```python
from build123d import *

# Parameters (mm, degrees)
PAD_DEPTH           = 110
PAD001_DEPTH        = 96
SKETCH003_W         = 118.6
SKETCH003_H         = 10
PAD002_DEPTH        = 3
PAD003_DEPTH        = 123
POCKET001_DEPTH     = 124.601
LINEARPATTERN_COUNT = 5
LINEARPATTERN_PITCH = 22.5
SKETCH012_W         = 6
SKETCH012_H         = 12
POCKET_DEPTH        = 5
SKETCH013_R         = 1.7
POCKET004_DEPTH     = 126.001
SKETCH014_R         = 7
SKETCH014_R_2       = 2
POCKET005_DEPTH     = 5


with BuildPart() as part:
    # Sketch → Pad (new body)
    with BuildSketch(Plane.XY):
        Polygon((62.3, 64.5), (-62.3, 64.5), (-62.3, -61.5), (-59.3, -61.5), (-59.3, 61.5), (59.3, 61.5), (59.3, -61.5), (62.3, -61.5), align=None)
    extrude(amount=PAD_DEPTH)

    # Sketch001 → Pad001 (join)
    with BuildSketch(Plane.XY):
        Polygon((-59.3, 59.5), (-57.3, 61.5), (-59.3, 61.5), align=None)
    pad001 = extrude(amount=PAD001_DEPTH)

    # Mirrored: Pad001 across YZ
    add(pad001.mirror(Plane.YZ))

    # Sketch003 (on DatumPlane) → Pad002 (join)
    with BuildSketch(Plane.XZ.offset(61.5)):
        with Locations((0, 5)):
            Rectangle(SKETCH003_W, SKETCH003_H)
    extrude(amount=-PAD002_DEPTH)

    # Sketch004 (on DatumPlane) → Pad003 (join)
    with BuildSketch(Plane.XZ.offset(61.5)):
        Polygon((-57.3, 117), (-59.3, 117), (-59.3, 100), (-57.3, 103), align=None)
        Polygon((57.3, 103), (57.3, 117), (59.3, 117), (59.3, 100), align=None)
    extrude(amount=-PAD003_DEPTH)

    # Sketch009 (on DatumPlane) → Pocket001 (cut, through all)
    with BuildSketch(Plane.YZ.offset(62.3)):
        with BuildLine():
            Line((-46, 20), (-46, 243))
            ThreePointArc((-42, 243), (-44, 245), (-46, 243))
            Line((-42, 243), (-42, 20))
            ThreePointArc((-46, 20), (-44, 18), (-42, 20))
        make_face()
    pocket001 = extrude(amount=-POCKET001_DEPTH, mode=Mode.SUBTRACT)

    # LinearPattern: Pocket001 ×5
    with Locations(*[(0, i * LINEARPATTERN_PITCH, 0) for i in range(1, LINEARPATTERN_COUNT)]):
        add(pocket001, mode=Mode.SUBTRACT)

    # Sketch012 (on DatumPlane) → Pocket (cut)
    with BuildSketch(Plane.YZ.offset(62.3)):
        with Locations((41.830656, 89.723986)):
            Rectangle(SKETCH012_W, SKETCH012_H)
        with Locations((41.830656, 62.651357)):
            Rectangle(SKETCH012_W, SKETCH012_H)
    extrude(amount=-POCKET_DEPTH, mode=Mode.SUBTRACT)

    # Sketch013 (on DatumPlane) → Pocket004 (cut, through all)
    with BuildSketch(Plane.XZ.offset(-64.5)):
        with Locations((20, 5)):
            Circle(SKETCH013_R)
        with Locations((-20, 5)):
            Circle(SKETCH013_R)
    extrude(amount=POCKET004_DEPTH, mode=Mode.SUBTRACT)

    # Sketch014 (on DatumPlane) → Pocket005 (cut)
    with BuildSketch(Plane.XZ.offset(-64.5)):
        with Locations((-16.307726, 38.976202)):
            Circle(SKETCH014_R)
        with Locations((-41.75, 38.976202)):
            Circle(SKETCH014_R)
        with Locations((-44.911871, 102.251883)):
            Circle(SKETCH014_R_2)
        Polygon((32, 0), (52, 0), (52, 18), (42, 28), (32, 18), align=None)
        Polygon((-52, 0), (-32, 0), (-32, 18), (-42, 28), (-52, 18), align=None)
    extrude(amount=POCKET005_DEPTH, mode=Mode.SUBTRACT)


with BuildPart() as part_1:
    # Body placement: moved
    add(part.part.moved(Location((1.4, 0, 0))))


solid = part_1.part
```
CAD build for the part. Positions are in the model's coordinates, mm. A direction names the side the tool comes from. Give positions to 0.01 mm unless a question says otherwise; leave off trailing zeros. Loops run counter-clockwise (first coordinate to the right, second up) from the corner with the lowest first, then second, coordinate; pieces in that order, holes last. Notation, with made-up numbers: (-2, -36.75) -> (25, -36.75) arc R26 ccw to (25, -15.75) -> close; hole circle Ø5 at (-35.75, 3). An arc over 180 degrees is marked (long way). Use a Markdown table: item, result.
1. Flat gauge pins, fed straight in: pin 1 (0.9 mm diameter, centred on x = -60, y = -13.5, fed in from +Z); pin 2 (1.5 mm diameter, centred on x = -7, y = -59.5, fed in from +Z); pin 3 (3 mm diameter, centred on x = -43.51, z = 102.25, fed in from +Y). Where does each tip first touch, or does it go through?
Check result:
| item | result |
|---|---|
| pin 1 | stops at z = 110 |
| pin 2 | stops at z = 10 |
| pin 3 | passes through |
2. Slice it at C-C (z = 5). Give the number of separate pieces and of enclosed holes in the cut face, plus the area to 3 significant figures.
Check result:
| item | result |
|---|---|
| separate pieces | 6 |
| enclosed holes | 0 |
| area | 1,310 mm^2 |
3. Slice it at D-D (x = -14). List the corners of the cut face in (y, z).
Check result:
| item | result |
|---|---|
| outline | (-61.5, 0) -> (-58.5, 0) -> (-58.5, 10) -> (-61.5, 10) -> close; (61.5, 0) -> (64.5, 0) -> (64.5, 32.04) -> (61.5, 32.04) -> close; (61.5, 45.92) -> (64.5, 45.92) -> (64.5, 110) -> (61.5, 110) -> close |
4. Slice it at A-A (y = 41). List the corners of the cut face in (x, z), plus the area to 3 significant figures.
Check result:
| item | result |
|---|---|
| outline | (-60.9, 0) -> (-57.9, 0) -> (-57.9, 100) -> (-55.9, 103) -> (-55.9, 117) -> (-57.9, 117) -> (-57.9, 110) -> (-60.9, 110) -> close; (58.7, 103) -> (60.7, 100) -> (60.7, 95.72) -> (63.7, 95.72) -> (63.7, 110) -> (60.7, 110) -> (60.7, 117) -> (58.7, 117) -> close; (60.7, 0) -> (63.7, 0) -> (63.7, 56.65) -> (60.7, 56.65) -> close; (60.7, 68.65) -> (63.7, 68.65) -> (63.7, 83.72) -> (60.7, 83.72) -> close |
| area | 650 mm^2 |
5. Which spindle directions (+Z, -Z, +X, -X, +Y, -Y) get a long thin tool onto all of the face, cutting with end or side? Do faces 4 (the flat face through (58.7, -54, 110)), 5 (the flat face through (-45.5, 63, 23.1)), 6 (the flat face through (58.7, -33, 110)), 7 (the flat face through (-57.9, 12, 114)), 8 (the flat face through (-59, -46, 68)). Say none if no direction does.
Check result:
| item | result |
|---|---|
| face 4 | +Z, -Y |
| face 5 | -Z, +Y, -Y |
| face 6 | +Z, -Z, -Y |
| face 7 | +Z, -X, +Y, -Y |
| face 8 | +Z, +X, -X |
6. Wall check: L1, parallel to X at y = -60.5, z = 5; L2, parallel to X at y = 63.9, z = 5; L3, parallel to Z at x = -18.6, y = -59.55. Give the ranges that are in metal, low to high. Write a range as [from, to].
Check result:
| item | result |
|---|---|
| L1 | x = [-60.9, -20.3], [-16.9, 19.7], [23.1, 63.7] |
| L2 | x = [-60.9, -50.6], [-30.6, -20.3], [-16.9, 19.7], [23.1, 33.4], [53.4, 63.7] |
| L3 | z = [0, 3.3], [6.7, 10] |
7. Mould opens along Y. For faces 1 (the flat face through (2, 64.5, 54)), 2 (the flat face through (-55.9, 55, 110)), 3 (the flat face through (-57.9, 13, 49)) say: pulls with the +Y half, pulls with the -Y half, needs draft (parallel to the pull), parting line crosses it, or undercut.
Check result:
| item | result |
|---|---|
| face 1 | pulls with the +Y half |
| face 2 | needs draft |
| face 3 | undercut |
8. Slice it at B-B (x = 4.5). List the corners of the cut face in (y, z).
Check result:
| item | result |
|---|---|
| outline | (-61.5, 0) -> (-58.5, 0) -> (-58.5, 10) -> (-61.5, 10) -> close; (61.5, 0) -> (64.5, 0) -> (64.5, 110) -> (61.5, 110) -> close |
